```python
from build123d import *

# Parameters (mm, degrees)
BOSS_EXTRUDE1_DEPTH           = 3
CSK_FOR_M3_SFHCS1_D           = 3.4
CSK_FOR_M3_SFHCS1_DEPTH       = 10
CSK_FOR_M3_SFHCS1_CSINK_D     = 6.72
CSK_FOR_M3_SFHCS1_CSINK_ANGLE = 90
CSK_FOR_M3_SFHCS1_TIP         = 1.021463052
FILLET1_R                     = 4


with BuildPart() as part:
    # Sketch1 → Boss-Extrude1 (new body)
    with BuildSketch(Plane(origin=(0, 0, 0), x_dir=(1, 0, 0), z_dir=(0, 1, 0))):
        with BuildLine():
            Line((-16.5, 20), (16.5, 20))
            Line((16.5, 20), (16.5, 0))
            Line((16.5, 0), (5.636918899, 0))
            ThreePointArc((5.636918899, 0), (4.479442445, 0.479442445), (4, 1.636918899))
            ThreePointArc((4, 1.636918899), (4.370899501, 3.526741264), (5.428571429, 5.13618996))
            ThreePointArc((5.428571429, 5.13618996), (6, 6.535898385), (5.428571429, 7.935606809))
            ThreePointArc((5.428571429, 7.935606809), (4.904567081, 8.902362767), (4.970825238, 10))
            Line((4.970825238, 10), (-4.970825238, 10))
            ThreePointArc((-4.970825238, 10), (-4.904567081, 8.902362767), (-5.428571429, 7.935606809))
            ThreePointArc((-5.428571429, 7.935606809), (-6, 6.535898385), (-5.428571429, 5.13618996))
            ThreePointArc((-5.428571429, 5.13618996), (-4.370899501, 3.526741264), (-4, 1.636918899))
            ThreePointArc((-4, 1.636918899), (-4.479442445, 0.479442445), (-5.636918899, 0))
            Line((-5.636918899, 0), (-16.5, 0))
            Line((-16.5, 0), (-16.5, 20))
        make_face()
    extrude(amount=BOSS_EXTRUDE1_DEPTH)

    # CSK for M3 SFHCS1
    with Locations(Plane(origin=(0, 3, 0), x_dir=(1, 0, 0), z_dir=(0, 1, 0))):
        with Locations((12.5, 16), (-12.5, 16)):
            CounterSinkHole(CSK_FOR_M3_SFHCS1_D / 2, CSK_FOR_M3_SFHCS1_CSINK_D / 2, depth=CSK_FOR_M3_SFHCS1_DEPTH, counter_sink_angle=CSK_FOR_M3_SFHCS1_CSINK_ANGLE)
            with Locations((0, 0, -(CSK_FOR_M3_SFHCS1_DEPTH + CSK_FOR_M3_SFHCS1_TIP / 2))):  # 118° drill point
                Cone(0, CSK_FOR_M3_SFHCS1_D / 2, CSK_FOR_M3_SFHCS1_TIP, mode=Mode.SUBTRACT)

    # Fillet1
    fillet1_edges = [part.edges().sort_by_distance(p)[0] for p in [
        (-16.5, 1.5, -20),
        (16.5, 1.5, -20),
    ]]
    fillet(fillet1_edges, radius=FILLET1_R)


solid = part.part
```
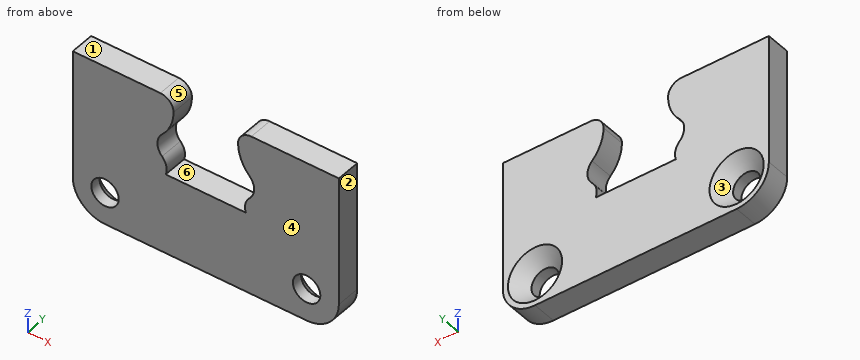
Input: part model. Units: mm. Frame: model coordinates. Face numbers are marked on the shaded views. A direction names the side the tool comes from. Give positions to 0.01 mm unless a question says otherwise; leave off trailing zeros. Write each loop counter-clockwise with the first axis right and the second up, starting at its lowest first coordinate (ties: lowest second). Pieces come first, ordered by that corner, then holes. Notation, with made-up numbers: (81, -12.75) - (119, -12.75) arc R21 cw to (119, 16.25) - close; hole circle Ø3 at (-18, -38). An arc over 180 degrees is marked (long way). Write item = value, one per line. Start each with the question number.
1. Ray query, L1, parallel to X at y = 0.75, z = -16; L2, parallel to Z at x = 12.5, y = 0.7; L3, parallel to X at y = 1.9, z = -17.5. Return the intervals inside material, ascending.
2. Section query B-B, the plane z = -2.5. Output: boundary loops of the cut face in (x, y).
3. Section query D-D, the plane y = 0.7. Output: boundary loops of the cut face in (x, z).
4. Access query for the marked faces 4, 5 and 6. Directions: +Z, -Z, +X, -X, +Y, -Y. A direction counts if a zero-diameter tool reaches every point of the face in a straight line with its end or side. Return the directions, or none.
5. First-contact query: pin 1 Ø1.5 at (x, y) = (2, 1) entering from +Z; pin 2 Ø4 at (x, z) = (12.5, -16) entering from +Y. Flat tips, straight axial feed; report the tip coordinate or a pass-through.
6. Section query C-C, the plane x = -1. Output: boundary loops of the cut face in (y, z), then the cut area to 3 significant figures.
7. Section query A-A, the plane y = 2.2. Output: boundary loops of the cut face in (x, z).
8. Mould query, pull axis X, two halves, no side actions, for the marked faces 1, 2 and 3. Classes: released by +X, released by -X, zero draft, split by the parting line, or undercut.
Check sheet entries:
q1.L1 = -16.5 to -14.2, -10.8 to 10.8, 14.2 to 16.5
q1.L2 = -20 to -17.7, -14.3 to 0
q1.L3 = -16.21 to -14.19, -10.81 to 10.81, 14.19 to 16.21
q2.outline = (-16.5, 0) - (-4.08, 0) - (-4.08, 3) - (-16.5, 3) - close; (4.08, 0) - (16.5, 0) - (16.5, 3) - (4.08, 3) - close
q3.outline = (-16.5, -16) arc R4 ccw to (-12.5, -20) - (12.5, -20) arc R4 ccw to (16.5, -16) - (16.5, 0) - (5.64, 0) arc R1.64 ccw to (4, -1.64) arc R5 ccw to (5.43, -5.14) arc R2 cw to (5.43, -7.94) arc R2 ccw to (4.97, -10) - (-4.97, -10) arc R2 ccw to (-5.43, -7.94) arc R2 cw to (-5.43, -5.14) arc R5 ccw to (-4, -1.64) arc R1.64 ccw to (-5.64, 0) - (-16.5, 0) - close; hole circle Ø3.4 at (-12.5, -16); hole circle Ø3.4 at (12.5, -16)
q4.face_4 = +Z, -Z, +X, -X, -Y
q4.face_5 = +Z, +Y, -Y
q4.face_6 = +Y, -Y
q5.pin_1 = -10
q5.pin_2 = 1.64
q6.outline = (0, -20) - (3, -20) - (3, -10) - (0, -10) - close
q6.area = 30.0 mm2
q7.outline = (-16.5, -16) arc R4 ccw to (-12.5, -20) - (12.5, -20) arc R4 ccw to (16.5, -16) - (16.5, 0) - (5.64, 0) arc R1.64 ccw to (4, -1.64) arc R5 ccw to (5.43, -5.14) arc R2 cw to (5.43, -7.94) arc R2 ccw to (4.97, -10) - (-4.97, -10) arc R2 ccw to (-5.43, -7.94) arc R2 cw to (-5.43, -5.14) arc R5 ccw to (-4, -1.64) arc R1.64 ccw to (-5.64, 0) - (-16.5, 0) - close; hole circle Ø5.12 at (-12.5, -16); hole circle Ø5.12 at (12.5, -16)
q8.face_1 = zero draft
q8.face_2 = released by +X
q8.face_3 = undercut
